from build123d import *

# Parameters (mm, degrees)
SKETCH1_W           = 45.72
SKETCH1_H           = 34.29
SKETCH1_R           = 3.175
BOSS_EXTRUDE1_DEPTH = 2.54
CUT_EXTRUDE1_DEPTH  = 2.54


with BuildPart() as part:
    # Sketch1 → Boss-Extrude1 (new body)
    with BuildSketch(Plane.XY):
        Rectangle(SKETCH1_W, SKETCH1_H)
        with Locations((15.24, 0.635)):
            Circle(SKETCH1_R, mode=Mode.SUBTRACT)
        with Locations(Location((-15.24, 0.635, 0), (0, 0, 180))):
            Circle(SKETCH1_R, mode=Mode.SUBTRACT)
    extrude(amount=BOSS_EXTRUDE1_DEPTH)

    # Sketch2 → Cut-Extrude1 (cut)
    with BuildSketch(Plane.XY):
        with BuildLine():
            Line((11.557, 0.635), (11.557, -17.145))
            Line((11.557, -17.145), (22.86, -17.145))
            Line((22.86, -17.145), (22.86, 0.635))
            Line((22.86, 0.635), (18.923, 0.635))
            ThreePointArc((18.923, 0.635), (15.24, 4.318), (11.557, 0.635))
        make_face()
        with BuildLine():
            Line((-11.557, 0.635), (-11.557, -17.145))
            Line((-11.557, -17.145), (-22.86, -17.145))
            Line((-22.86, -17.145), (-22.86, 0.635))
            Line((-22.86, 0.635), (-18.923, 0.635))
            ThreePointArc((-18.923, 0.635), (-15.24, 4.318), (-11.557, 0.635))
        make_face()
    extrude(amount=CUT_EXTRUDE1_DEPTH, mode=Mode.SUBTRACT)


solid = part.part
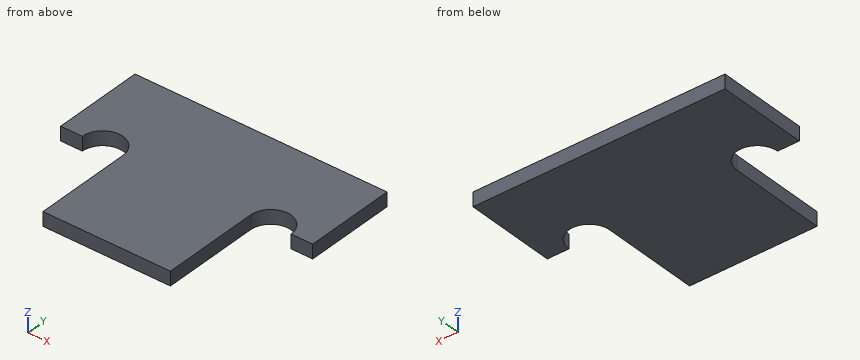
Could you check a few things on this model? Use its own coordinates, in mm. Round coordinates to 2 decimals unless told otherwise and drop trailing zeros. Order: outer loops, then holes, each group sorted by start corner. A loop starts at its lowest first (then second) coordinate and runs counter-clockwise, first axis right, second up.
Q1. Imagine slicing it at B-B, the plane x = 15.24. List the corners of the cut face in (y, z) for me (3 decimals).
Geometry says:
outline: (4.318, 0) - (17.145, 0) - (17.145, 2.54) - (4.318, 2.54) - close
Q2. I'm going to push flat-ended pins straight in: P1, Ø1.3, axis at y = -11.5, z = 1.5, coming from the -X side; P2, Ø0.8, axis at y = -5, z = 1, coming from the +X side; P3, Ø1.5, axis at x = 12, z = 0.5, coming from the -Y side (3 decimals). Where does each tip first touch, or does it pass through?
Geometry says:
P1: stops at x = -11.56
P2: stops at x = 11.56
P3: stops at y = -17.145
Q3. Imagine slicing it at A-A, the plane z = 1.15. List the corners of the cut face in (x, y) for me (3 decimals), then the cut area to 3 significant figures.
Geometry says:
outline: (-22.86, 0.635) - (-18.923, 0.635) arc R3.683 cw to (-11.557, 0.635) - (-11.557, -17.145) - (11.557, -17.145) - (11.557, 0.635) arc R3.683 cw to (18.923, 0.635) - (22.86, 0.635) - (22.86, 17.145) - (-22.86, 17.145) - close
area: 1,120 mm2
Q4. Imagine slicing it at C-C, the plane y = -13.5. List the corners of the cut face in (x, z) for me, then the cut area to 3 significant figures.
Geometry says:
outline: (-11.56, 0) - (11.56, 0) - (11.56, 2.54) - (-11.56, 2.54) - close
area: 58.7 mm2
Q5. Please list where these lines run through material, in increasing order: probe 1 along X at (y, z) = (3, 1.65); probe 2 along X at (y, z) = (-9, 1.6); probe 3 along X at (y, z) = (1, 1.85).
Geometry says:
probe 1: x = -22.86 to -18.06, -12.42 to 12.42, 18.06 to 22.86
probe 2: x = -11.56 to 11.56
probe 3: x = -22.86 to -18.9, -11.58 to 11.58, 18.9 to 22.86
